Verification items for this drawing (mm, ordinates from the low corner). A direction names the side the tool comes from. Coordinates: 2 decimals unless noted, no trailing zeros. Write each loop counter-clockwise with the first axis right and the second up, starting at its lowest first coordinate (ties: lowest second). Pieces come first, ordered by that corner, then holes. Notation, with made-up numbers: M 12,42.25 L 26,42.25 A18 ccw 26,63.25 Z; hole C -26,2.25 d3. An arc over 180 degrees is marked long. Write each question's results on one line, items separated by ' | '.
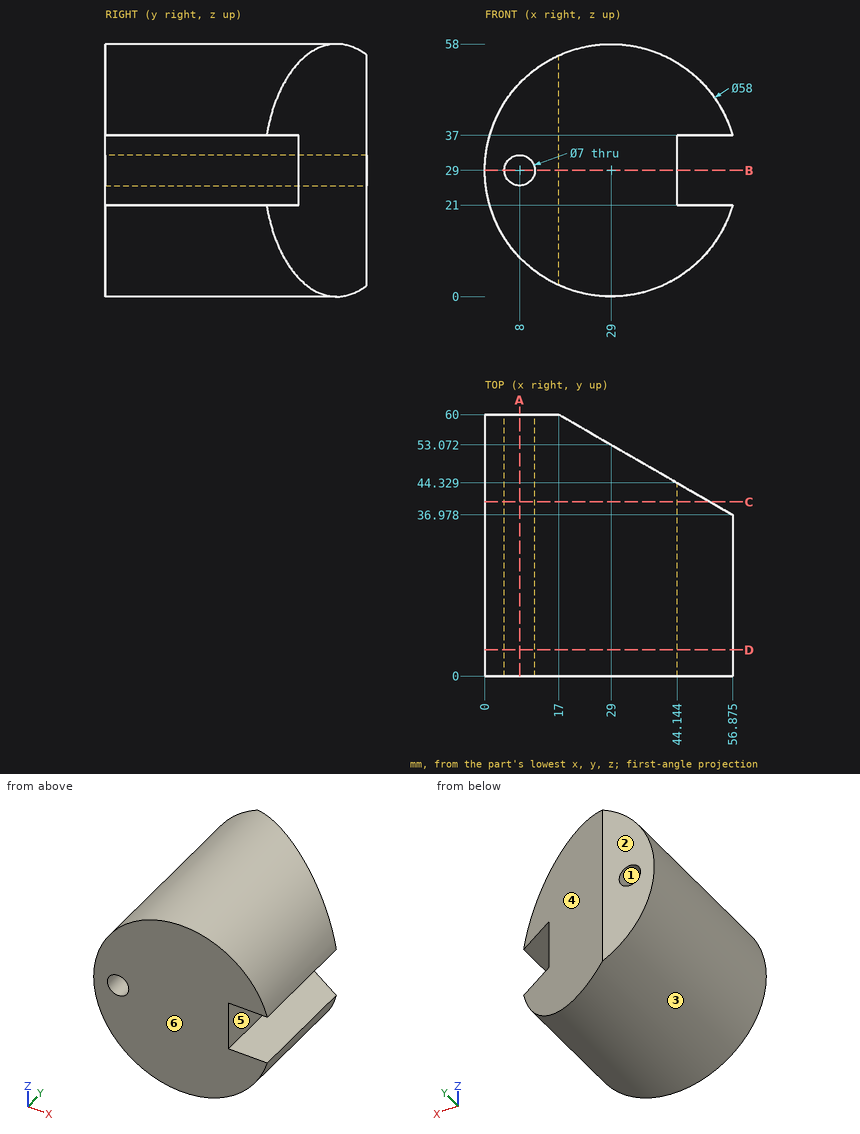
Q1. Access from +Z, -Z, +X, -X, +Y, -Y to the whole of each face (thin tool, end or side, straight path). Record for the marked faces 5 and 6.
Geometry check:
face 5: +X, +Y, -Y | face 6: +Z, -Z, +X, -X, -Y
Q2. Mould release check, pull along X, two halves, no side actions. Record for the marked faces 1, 2, 3 and 4: pulls with the +X half, pulls with the -X half, needs draft (parallel to the pull), parting line crosses it, or undercut.
Geometry check:
face 1: undercut | face 2: needs draft | face 3: parting line crosses it | face 4: pulls with the +X half
Q3. Depth check by flat-ended pin: P1, Ø12, axis at x = 14, z = 51, coming from the -Y side; P2, Ø6, axis at x = 41, y = 24.5, coming from the +Z side; P3, Ø3, axis at y = 11, z = 51, coming from the +X side; P4, Ø1.5, axis at x = 7.5, y = 6, coming from the +Z side. Enter the tip coordinate at first touch or a pass-through.
Geometry check:
P1: stops at y = 0 | P2: stops at z = 56.57 | P3: stops at x = 49.51 | P4: stops at z = 49.26
Q4. Sectioned sample at A-A on x = 8. Record the cut outline in (y, z), and give its area (3 significant figures).
Geometry check:
outline: M 0,9 L 60,9 L 60,25.5 L 0,25.5 Z; M 0,32.5 L 60,32.5 L 60,49 L 0,49 Z | area: 1,980 mm2
Q5. Sectioned sample at D-D on y = 6. Record the cut outline in (x, z) (1 decimal).
Geometry check:
outline: M 44.1,21 L 44.1,37 L 56.9,37 A29 ccw long 56.9,21 Z; hole C 8,29 d7
Q6. Sectioned sample at C-C on y = 40. Record the cut outline in (x, z), and give its area (3 significant figures).
Geometry check:
outline: M 44.14,21 L 44.14,37 L 51.64,37 L 51.64,47.12 A29 ccw long 51.64,10.88 L 51.64,21 Z; hole C 8,29 d7 | area: 2,330 mm2
Q7. Scan lines: probe 1 along X at (y, z) = (12, 29); probe 2 along Z at (x, y) = (29.5, 24.5) (1 decimal); probe 3 along Z at (x, y) = (52.5, 21.5) (1 decimal). Record each from-to range of solid material in increasing order.
Geometry check:
probe 1: x = 0 to 4.5, 11.5 to 44.14 | probe 2: z = 0 to 58 | probe 3: z = 12 to 21, 37 to 46
Q8. Sectioned sample at B-B on z = 29. Record the cut outline in (x, y).
Geometry check:
outline: M 0,0 L 4.5,0 L 4.5,60 L 0,60 Z; M 11.5,0 L 44.14,0 L 44.14,44.33 L 17,60 L 11.5,60 Z
